Part model, mm, in its own coordinate system. A direction names the side the tool comes from. Coordinates: 2 decimals unless noted, no trailing zeros. Order: outer loops, then holes, each group sorted by start corner. A loop starts at its lowest first (then second) coordinate and runs counter-clockwise, first axis right, second up.
1) Cut at C-C (x = 61.5). List the corners of the cut face in (y, z).
2) Mould opens along X. For faces 3 (the flat face through (10, 70, 2)), 4 (the flat face through (0, 35, 2)), 5 (the cylindrical face through (9.609, 64.474, 2.028)) say: +X half, -X half, draft (parallel to the pull), parting line (faces both ways), or undercut.
3) Cut at B-B (z = 2.8). List the corners of the cut face in (x, y).
4) Pin check, flat tips, straight feed: pin 1 Ø5.5 at (x, y) = (10, 61.5) entering from -Z (3 decimals); pin 2 Ø1.5 at (y, z) = (33, 0.5) entering from +X; pin 3 Ø1 at (y, z) = (28, 1.5) entering from +X; pin 4 Ø1 at (x, z) = (59.5, 1.5) entering from +Y. Stop position of each tip, or through.
5) Tool access for faces 1 (the flat face through (19, 28, 0)), 2 (the cylindrical face through (21, 22, 2)): list every direction of +Z, -Z, +X, -X, +Y, -Y with a clear straight run to the whole face (end or side of a thin tool).
6) Cut at A-A (y = 10). List the corners of the cut face in (x, z), and give its area (3 significant figures).
7) Wall check: L1, parallel to Y at x = 10, z = 1.25; L2, parallel to Y at x = 8.5, z = 1; L3, parallel to X at y = 43.5, z = 0.45. Give the ranges that are in metal, low to high.
```python
from build123d import *

# Parameters (mm, degrees)
PAD_DEPTH       = 4
POCKET_DEPTH    = 4.001
SKETCH002_R     = 3
POCKET001_DEPTH = 4.001
FILLET_R        = 5
FILLET001_R     = 0.5


with BuildPart() as part:
    # Sketch → Pad (new body)
    with BuildSketch(Plane.XY):
        with BuildLine():
            Line((0, 0), (70, 0))
            Line((70, 0), (70, 20))
            ThreePointArc((20, 70), (37.928932, 37.928932), (70, 20))
            Line((20, 70), (0, 70))
            Line((0, 70), (0, 0))
        make_face()
    extrude(amount=PAD_DEPTH)

    # Sketch001 → Pocket (cut, through all)
    with BuildSketch(Plane.XY.offset(4)):
        with BuildLine():
            ThreePointArc((20, 54.914649), (34.393398, 34.393398), (54.914649, 20))
            Line((20, 20), (54.914649, 20))
            Line((20, 54.914649), (20, 20))
        make_face()
    extrude(amount=-POCKET_DEPTH, mode=Mode.SUBTRACT)

    # Sketch002 → Pocket001 (cut, through all)
    with BuildSketch(Plane.XY.offset(4)):
        with Locations((10, 28.5)):
            Circle(SKETCH002_R)
        with Locations((10, 61.5)):
            Circle(SKETCH002_R)
        with Locations((28.5, 10)):
            Circle(SKETCH002_R)
        with Locations((61.5, 10)):
            Circle(SKETCH002_R)
    extrude(amount=-POCKET001_DEPTH, mode=Mode.SUBTRACT)

    # Fillet
    fillet_edges = [part.edges().sort_by_distance(p)[0] for p in [
        (20, 20, 2),
    ]]
    fillet(fillet_edges, radius=FILLET_R)

    # Fillet001
    fillet001_edges = [part.edges().sort_by_distance(p)[0] for p in [
        (20, 54.914649, 2),
        (54.914649, 20, 2),
    ]]
    fillet(fillet001_edges, radius=FILLET001_R)


solid = part.part
```
Geometry check:
1. outline: (0, 0) - (7, 0) - (7, 4) - (0, 4) - close; (13, 0) - (22.63, 0) - (22.63, 4) - (13, 4) - close
2. face 3: draft
2. face 4: -X half
2. face 5: undercut
3. outline: (0, 0) - (70, 0) - (70, 20) arc R67.5 cw to (20, 70) - (0, 70) - close; hole circle Ø6 at (10, 28.5); hole circle Ø6 at (10, 61.5); hole (20, 25) arc R5 ccw to (25, 20) - (52.74, 20) arc R0.5 ccw to (52.97, 20.95) arc R72.5 cw to (20.95, 52.97) arc R0.5 ccw to (20, 52.74) - close; hole circle Ø6 at (28.5, 10); hole circle Ø6 at (61.5, 10)
4. pin 1: passes through
4. pin 2: stops at x = 44.38
4. pin 3: stops at x = 51.4
4. pin 4: stops at y = 23.65
5. face 1: -Z, +X, -X, +Y, -Y
5. face 2: +Z, -Z
6. outline: (0, 0) - (25.5, 0) - (25.5, 4) - (0, 4) - close; (31.5, 0) - (58.5, 0) - (58.5, 4) - (31.5, 4) - close; (64.5, 0) - (70, 0) - (70, 4) - (64.5, 4) - close
6. area: 232 mm2
7. L1: y = 0 to 25.5, 31.5 to 58.5, 64.5 to 70
7. L2: y = 0 to 25.9, 31.1 to 58.9, 64.1 to 70
7. L3: x = 0 to 20, 26.68 to 32.94
